Autodesk Inventor part; units mm, degrees
ref_plane "YZ Plane" through (0, 0, 0) normal (1, 0, 0) x (0, 1, 0)
ref_plane "XZ Plane" through (0, 0, 0) normal (0, 1, 0) x (-1, 0, 0)
ref_plane "XY Plane" through (0, 0, 0) normal (0, 0, 1) x (1, 0, 0)
sketch "Sketch1" plane through (0, 0, 0) normal (0, 0, 1) x (1, 0, 0)
  arc A0 (78, -128.1249) -> (-78, -128.1249) centre (0, 0) ccw
  line L0 (78, -128.1249) -> (78, -270)
  line L1 (78, -270) -> (-78, -270)
  line L2 (-78, -270) -> (-78, -128.1249)
  line L3 (-78, -30) -> (78, -270) construction
  line L4 (78, -30) -> (-78, -270) construction
extrude "Extrusion1" add sketch "Sketch1" along normal blind 80
sketch "Sketch2" plane through (0, 0, 80) normal (0, 0, 1) x (1, 0, 0)
  circle A0 centre (0, 0) radius 20
extrude "Extrusion2" cut sketch "Sketch2" against normal through all
sketch "Sketch3" plane through (0, 0, 80) normal (0, 0, 1) x (1, 0, 0)
  circle A0 centre (0, 0) radius 32
sketch "Sketch4" plane through (0, 0, 80) normal (0, 0, 1) x (1, 0, 0)
  circle A0 centre (0, 0) radius 20
extrude "Extrusion3" add sketch "Sketch3" along normal blind 8
extrude "Extrusion4" cut sketch "Sketch4" along normal blind 8
properties part number "BigCounterWeight"
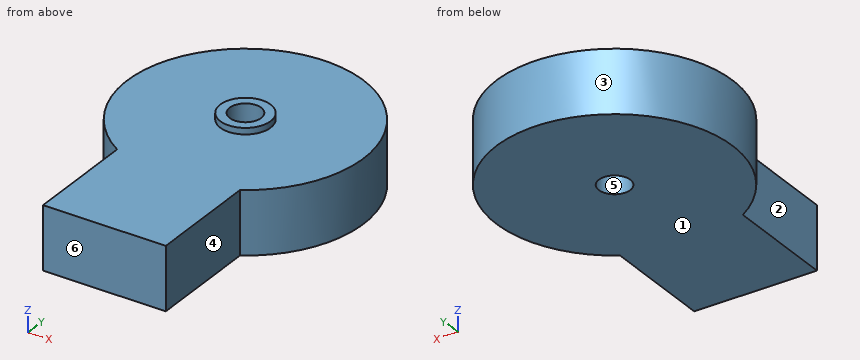
Geometry check sheet. Reference: the model listing, model coordinates, mm. Face numbers are marked on the shaded views. A direction names the side the tool comes from. Coordinates: 2 decimals unless noted, no trailing zeros. Write each loop counter-clockwise with the first axis right and the second up, starting at its lowest first coordinate (ties: lowest second). Pieces come first, ordered by that corner, then holes. Notation, with made-up numbers: M 63,7 L 95,7 A23 cw 95,46 Z; hole C 86,78.5 d2. An arc over 180 degrees is marked long. Use one line per item in the form item = value. Start each with the question number.
1) Release check for a two-part mould opening along X. For the marked faces 3, 4, 5 and 6 record: pulls with the +X half, pulls with the -X half, needs draft (parallel to the pull), parting line crosses it, or undercut.
2) Thickness scan on probe 1 along Y at (x, z) = (0, 51); probe 2 along Z at (x, y) = (-47.5, -44); probe 3 along X at (y, z) = (-2.5, 67.5). Record the ranges inside material, lowest first. Write a range as from..to.
3) Section check B-B on y = 0. Enter the section's corners in (x, z).
4) Section check C-C on z = 14. Enter the section's corners in (x, y), and give its area (3 significant figures).
5) Section check A-A on x = 0. Enter the section's corners in (y, z).
6) Go/stop test with flat-tipped pins: pin 1 Ø12 at (x, z) = (-41.5, 29.5) entering from +Y; pin 2 Ø1.5 at (y, z) = (12.5, 49) entering from +X; pin 3 Ø3 at (x, z) = (7.5, 30.5) entering from +Y. Record where each tip stops, or that it passes through.
7) Section check D-D on x = -114. Enter the section's corners in (y, z).
8) Set-up check for the marked faces 1 and 2: record each of +Z, -Z, +X, -X, +Y, -Y from which the full face is reachable in a straight line by a thin tool's end or side.
Responses:
q1.face_3 = parting line crosses it
q1.face_4 = pulls with the +X half
q1.face_5 = undercut
q1.face_6 = needs draft
q2.probe_1 = -270..-20, 20..150
q2.probe_2 = 0..80
q2.probe_3 = -149.98..-19.84, 19.84..149.98
q3.outline = M -150,0 L -20,0 L -20,88 L -32,88 L -32,80 L -150,80 Z; M 20,0 L 150,0 L 150,80 L 32,80 L 32,88 L 20,88 Z
q4.outline = M -78,-270 L 78,-270 L 78,-128.12 A150 ccw long -78,-128.12 Z; hole C 0,0 d40
q4.area = 89,300 mm2
q5.outline = M -270,0 L -20,0 L -20,88 L -32,88 L -32,80 L -270,80 Z; M 20,0 L 150,0 L 150,80 L 32,80 L 32,88 L 20,88 Z
q6.pin_1 = 145.74
q6.pin_2 = 149.54
q6.pin_3 = 149.88
q7.outline = M -97.49,0 L 97.49,0 L 97.49,80 L -97.49,80 Z
q8.face_1 = -Z, +X, -X, +Y, -Y
q8.face_2 = +Z, -Z, -X, -Y
